Source: three-view drawing plus pictorial views. Frame: mm from the lowest corner of the part. A direction names the side the tool comes from. Round coordinates to 2 decimals unless told otherwise and drop trailing zeros. Loops run counter-clockwise (first coordinate to the right, second up) from the corner with the lowest first, then second, coordinate; pieces in that order, holes last. Notation, with made-up numbers: (30, -27.5) -> (64, -27.5) arc R10 ccw to (64, -21.5) -> close; hole circle Ø6 at (-12.5, 85). An arc over 180 degrees is marked (long way). Answer in a Markdown table with one row per item.
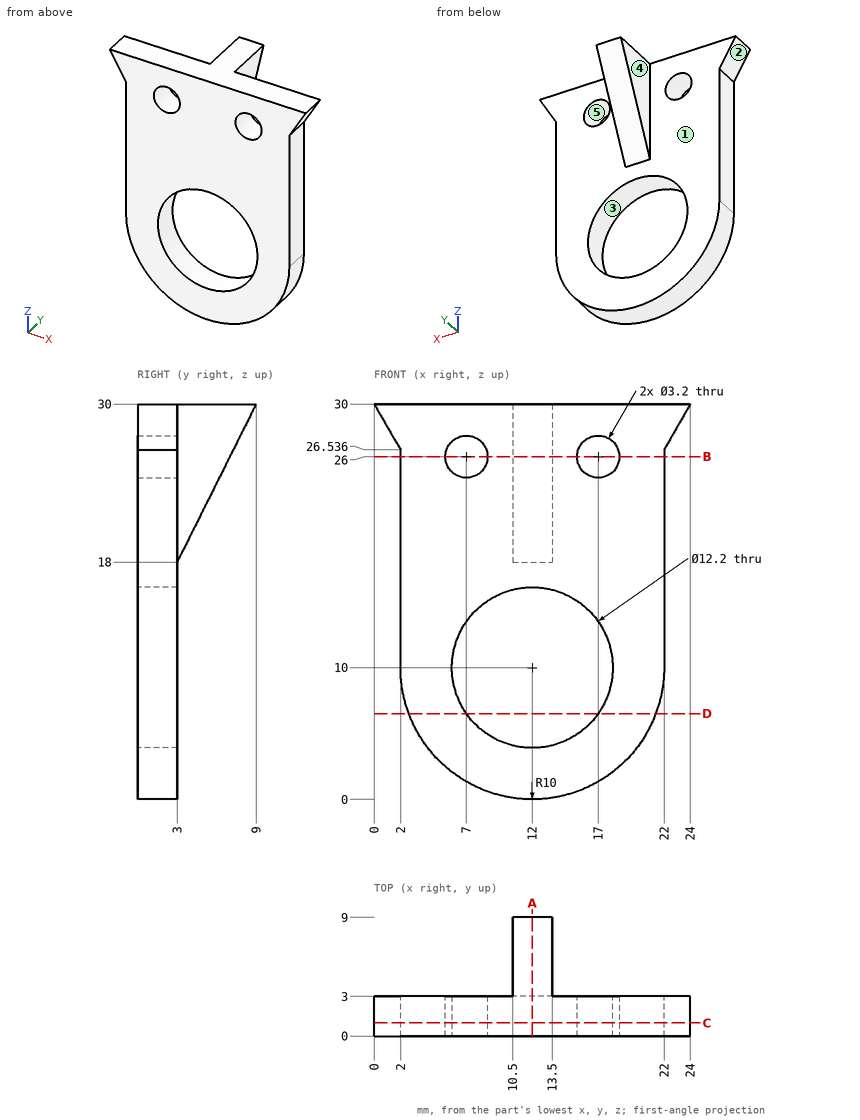
Item 1: Reachability of the marked faces 4 and 5 from +Z, -Z, +X, -X, +Y, -Y: full face, straight path, thin tool, end or side. Return the list, or none.
Answer:
| item | result |
|---|---|
| face 4 | +Z, -Z, -X, +Y |
| face 5 | +Y, -Y |
Item 2: Line query: probe 1 along X at (y, z) = (2.2, 26); probe 2 along X at (y, z) = (2.45, 10); probe 3 along Z at (x, y) = (12, 1.55). Output: solid intervals per line, ascending. Write a range as [from, to].
Answer:
| item | result |
|---|---|
| probe 1 | x = [2, 5.4], [8.6, 15.4], [18.6, 22] |
| probe 2 | x = [2, 5.9], [18.1, 22] |
| probe 3 | z = [0, 3.9], [16.1, 30] |
Item 3: Cut plane B-B (z = 26). Output: boundary loops of the cut face in (x, y), then the cut area to 3 significant figures.
Answer:
| item | result |
|---|---|
| outline | (2, 0) -> (5.4, 0) -> (5.4, 3) -> (2, 3) -> close; (8.6, 0) -> (15.4, 0) -> (15.4, 3) -> (13.5, 3) -> (13.5, 7) -> (10.5, 7) -> (10.5, 3) -> (8.6, 3) -> close; (18.6, 0) -> (22, 0) -> (22, 3) -> (18.6, 3) -> close |
| area | 52.8 mm² |
Item 4: Cut plane A-A (x = 12). Output: boundary loops of the cut face in (y, z).
Answer:
| item | result |
|---|---|
| outline | (0, 0) -> (3, 0) -> (3, 3.9) -> (0, 3.9) -> close; (0, 16.1) -> (3, 16.1) -> (3, 18) -> (9, 30) -> (0, 30) -> close |
Item 5: Cut plane C-C (y = 1). Output: boundary loops of the cut face in (x, z), then the cut area to 3 significant figures.
Answer:
| item | result |
|---|---|
| outline | (0, 30) -> (2, 26.54) -> (2, 10) arc R10 ccw to (22, 10) -> (22, 26.54) -> (24, 30) -> close; hole circle Ø3.2 at (7, 26); hole circle Ø12.2 at (12, 10); hole circle Ø3.2 at (17, 26) |
| area | 431 mm² |
Item 6: Pin query (flat end, axial travel): pin 1 Ø5 at (y, z) = (6, 26) entering from -X; pin 2 Ø7 at (x, z) = (6.5, 15.5) entering from +Y; pin 3 Ø2.5 at (y, z) = (1.5, 16.5) entering from +X. Return the tip coordinate at first contact, or that it passes through.
Answer:
| item | result |
|---|---|
| pin 1 | stops at x = 10.5 |
| pin 2 | stops at y = 3 |
| pin 3 | stops at x = 22 |
Item 7: Cut plane D-D (z = 6.5). Output: boundary loops of the cut face in (x, y), then the cut area to 3 significant figures.
Answer:
| item | result |
|---|---|
| outline | (2.63, 0) -> (7, 0) -> (7, 3) -> (2.63, 3) -> close; (17, 0) -> (21.37, 0) -> (21.37, 3) -> (17, 3) -> close |
| area | 26.2 mm² |
Item 8: Draft query along Z for the marked faces 1, 2 and 3. Return one class per face: pulls with the +Z half, pulls with the -Z half, needs draft (parallel to the pull), parting line crosses it, or undercut.
Answer:
| item | result |
|---|---|
| face 1 | needs draft |
| face 2 | pulls with the -Z half |
| face 3 | undercut |
